Geometry: final body of the model. Coordinates: model frame, mm. Face numbers are marked on the shaded views. A direction names the side the tool comes from. Give positions to 0.01 mm unless a question says otherwise; leave off trailing zeros. Write each loop counter-clockwise with the first axis right and the second up, starting at its lowest first coordinate (ties: lowest second). Pieces come first, ordered by that corner, then holes.
Q1. Line query: L1, parallel to Z at x = 0.5, y = -7.25; L2, parallel to Y at x = 1, z = 12.25; L3, parallel to X at y = -3.75, z = -2.25. Output: solid intervals per line, ascending.
Q2. Pin query (flat end, axial travel): pin 1 (3 mm diameter, centred on x = 0, y = -8.5, fed in from +Z); pin 2 (2 mm diameter, centred on x = 3, z = 2.5, fed in from +Y); pin 3 (2 mm diameter, centred on y = -7, z = -8, fed in from +X). Return the tip coordinate at first contact, or that it passes through.
Q3. Cut plane B-B on z = 7.25. Return the cut outline in (x, y), plus the area to 3 significant figures.
Q4. Cut plane C-C on y = -7.5. Return the cut outline in (x, z).
Q5. Reachability of the marked faces 1 and 2 from +Z, -Z, +X, -X, +Y, -Y: full face, straight path, thin tool, end or side. Return the list, or none.
Q6. Cut plane A-A on x = 0. Return the cut outline in (y, z).
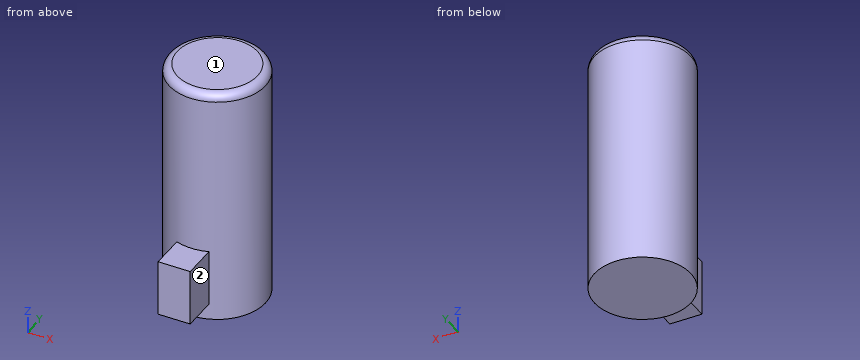
Solid Edge part; units mm, degrees
sketch "Sketch1" plane through (0, 0, 0) normal (0, 0, 1) x (1, 0, 0)
  circle A0 centre (0, 0) radius 6
extrude "Protrusion1" add sketch "Sketch1" along normal mid plane 30
sketch "Sketch2" plane through (0, 0, 0) normal (0, -1, 0) x (1, 0, 0)
  line L0 (2, -13) -> (-2, -13)
  line L1 (-2, -13) -> (-2, -6)
  line L2 (-2, -6) -> (2, -6)
  line L3 (2, -6) -> (2, -13)
extrude "ExtrudedProtrusion_2" add sketch "Sketch2" along normal blind 10
fillet "Round_1" radius 1 1 edges at (-6, 0, 15)
properties material "PVC"
Data:
1. L1: z = -13 to -6
1. L2: y = -5.92 to 5.92
1. L3: x = -4.68 to 4.68
2. pin 1: stops at z = -6
2. pin 2: stops at y = 5.66
2. pin 3: stops at x = 2
3. outline: circle Ø12 at (0, 0)
3. area: 113 mm2
4. outline: (-2, -13) - (2, -13) - (2, -6) - (-2, -6) - close
5. face 1: +Z, +X, -X, +Y, -Y
5. face 2: +Z, -Z, +X, -Y
6. outline: (-10, -13) - (-6, -13) - (-6, -15) - (6, -15) - (6, 14) arc R1 ccw to (5, 15) - (-5, 15) arc R1 ccw to (-6, 14) - (-6, -6) - (-10, -6) - close
